from build123d import *

# Parameters (mm, degrees)
BOSS_EXTRUDE1_DEPTH = 1.5875


with BuildPart() as part:
    # Sketch1 → Boss-Extrude1 (new body, symmetric)
    with BuildSketch(Plane(origin=(0, 0, 0), x_dir=(1, 0, 0), z_dir=(0, 1, 0))):
        Polygon((-9.525, 6.35), (-9.525, -6.35), (-6.35, -6.35), (-6.35, -9.525), (6.35, -9.525), (6.35, -6.35), (9.525, -6.35), (9.525, 6.35), (6.35, 6.35), (6.35, 9.525), (-6.35, 9.525), (-6.35, 6.35), align=None)
    extrude(amount=BOSS_EXTRUDE1_DEPTH, both=True)


solid = part.part
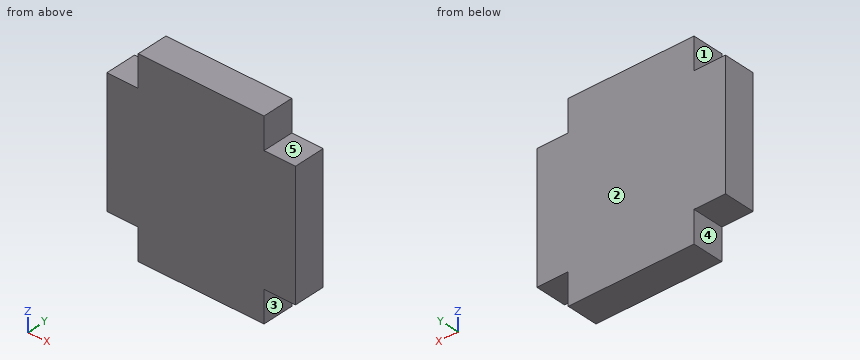
The listing builds one solid part. Answer for the finished solid, in the listing's coordinates (mm). Face numbers are marked on the shaded views. A direction names the side the tool comes from. Round coordinates to 2 decimals unless told otherwise and drop trailing zeros. Order: outer loops, then holes, each group sorted by start corner. A loop starts at its lowest first (then second) coordinate and runs counter-clockwise, first axis right, second up. Notation, with made-up numbers: (82.5, -32) - (108.5, -32) arc R21 ccw to (108.5, -11) - close; hole circle Ø7 at (36, 54.5). An arc over 180 degrees is marked (long way). Write item = value, one per line. Start each with the question number.
1) Section B-B, the plane z = -7 is taken. Write down the section's boundary in (x, y), plus the area to 3 significant figures.
2) Section A-A, the plane y = 0.15 is taken. Write down the section's boundary in (x, z) (3 decimals), plus the area to 3 significant figures.
3) A straight line is drawn through the part: L1, parallel to Z at x = -7.5, y = 0.85. Find the intervals that lie inside material, in ascending order.
4) Given pin 1 (1.6 mm diameter, centred on y = -0.5, z = -8.5, fed in from -X); pin 2 (1.6 mm diameter, centred on x = 8.5, y = 0, fed in from -Z); pin 3 (1 mm diameter, centred on x = 8.5, y = 0, fed in from +Z), each flat-ended and moving along its own axis, determine where each tip first touches the part or whether it passes through.
5) For the marked faces 1, 2, 3, 4 and 5, determine the directions among +Z, -Z, +X, -X, +Y, -Y from which every point of the face is accessible in a straight line to the end or side of a thin tool.
Results list:
q1.outline = (-6.35, -1.59) - (6.35, -1.59) - (6.35, 1.59) - (-6.35, 1.59) - close
q1.area = 40.3 mm^2
q2.outline = (-9.525, -6.35) - (-6.35, -6.35) - (-6.35, -9.525) - (6.35, -9.525) - (6.35, -6.35) - (9.525, -6.35) - (9.525, 6.35) - (6.35, 6.35) - (6.35, 9.525) - (-6.35, 9.525) - (-6.35, 6.35) - (-9.525, 6.35) - close
q2.area = 323 mm^2
q3.L1 = -6.35 to 6.35
q4.pin_1 = -6.35
q4.pin_2 = -6.35
q4.pin_3 = 6.35
q5.face_1 = +Z, -X, +Y, -Y
q5.face_2 = +Z, -Z, +X, -X, +Y
q5.face_3 = -Z, +X, +Y, -Y
q5.face_4 = -Z, -X, +Y, -Y
q5.face_5 = +Z, +X, +Y, -Y
